The listing builds one solid part. Answer for the finished solid, in the listing's coordinates (mm). Face numbers are marked on the shaded views. Coordinates: 2 decimals unless noted, no trailing zeros. Order: outer loops, then holes, each group sorted by start corner. A loop starts at its lowest first (then second) coordinate and runs counter-clockwise, first axis right, second up. Notation, with made-up numbers: (-4, 56) -> (39, 56) arc R27 ccw to (39, 95) -> close; hole circle Ø9 at (-18.5, 52). An arc over 180 degrees is marked (long way). Answer in a Markdown table with one row per item.
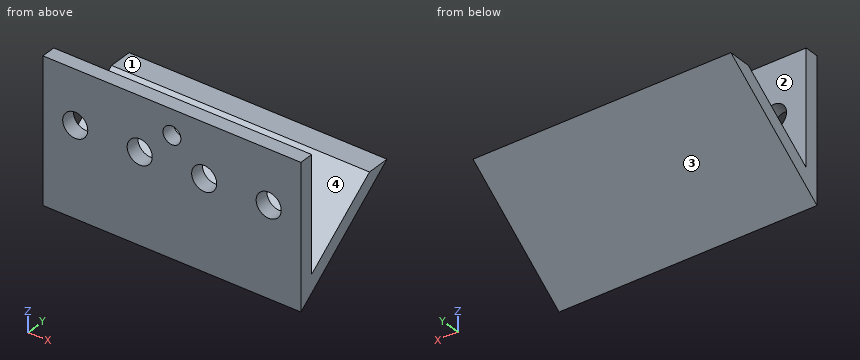
```python
from build123d import *

# Parameters (mm, degrees)
F0_W     = 72
F0_H     = 40
F0_R     = 3.5
F0_R_2   = 2.5
F1_DEPTH = 4
F3_DEPTH = 72
F5_DEPTH = 72


with BuildPart() as f1:
    # F0 (on Front) → F1 (new body)
    with BuildSketch(Plane.XZ):
        with Locations((0, -5)):
            Rectangle(F0_W, F0_H)
        with Locations((-27, 0)):
            Circle(F0_R, mode=Mode.SUBTRACT)
        with Locations((-9, 0)):
            Circle(F0_R, mode=Mode.SUBTRACT)
        with Locations((9, 0)):
            Circle(F0_R, mode=Mode.SUBTRACT)
        with Locations((27, 0)):
            Circle(F0_R, mode=Mode.SUBTRACT)
        with Locations((0, 8)):
            Circle(F0_R_2, mode=Mode.SUBTRACT)
    extrude(amount=F1_DEPTH)

    # F2 (on face) → F3 (cut)
    with BuildSketch(Plane.YZ.offset(36)):
        Polygon((0, -22), (-4, -25), (0, -25), align=None)
    extrude(amount=-F3_DEPTH, mode=Mode.SUBTRACT)

    # F4 (on face) → F5 (join)
    with BuildSketch(Plane.YZ.offset(36)):
        Polygon((0, -17), (0, -22), (28, -1), (21.5, -1), align=None)
    extrude(amount=-F5_DEPTH)


solid = f1.part
```
(1) A cutting plane is placed at A-A, the plane x = 0. Determine the outline of the cut face in (y, z), then the cut area to 3 significant figures.
Check values:
| item | result |
|---|---|
| outline | (-4, -25) -> (28, -1) -> (21.5, -1) -> (0, -17) -> (0, 5.5) -> (-4, 5.5) -> close; (-4, 10.5) -> (0, 10.5) -> (0, 15) -> (-4, 15) -> close |
| area | 256 mm² |
(2) Find the intervals of material crossed by line 1 along Y through (x, z) = (-24.5, 5); line 2 along Z through (x, y) = (27, -1); line 3 along Y through (x, z) = (6, -14), in increasing order. Write a range as from..to.
Check values:
| item | result |
|---|---|
| line 1 | -4..0 |
| line 2 | -22.75..-3.5, 3.5..15 |
| line 3 | -4..0, 4.03..10.67 |
(3) Flat-ended cylindrical pins translate along their axes: pin 1 (2 mm diameter, centred on x = 9, y = 16, fed in from +Z); pin 2 (9 mm diameter, centred on x = 27, z = 0, fed in from -Y); pin 3 (7 mm diameter, centred on x = -16, y = 26, fed in from +Z); pin 4 (8 mm diameter, centred on x = -17, y = 10, fed in from -Z). Find the tip coordinate at first contact, or state that the pin passes through.
Check values:
| item | result |
|---|---|
| pin 1 | z = -4.35 |
| pin 2 | y = -4 |
| pin 3 | z = -1 |
| pin 4 | z = -17.5 |
(4) A cutting plane is placed at C-C, the plane z = 8. Determine the outline of the cut face in (x, y), then the cut area to 3 significant figures.
Check values:
| item | result |
|---|---|
| outline | (-36, -4) -> (-2.5, -4) -> (-2.5, 0) -> (-36, 0) -> close; (2.5, -4) -> (36, -4) -> (36, 0) -> (2.5, 0) -> close |
| area | 268 mm² |
(5) A cutting plane is placed at D-D, the plane x = 27. Determine the outline of the cut face in (y, z).
Check values:
| item | result |
|---|---|
| outline | (-4, -25) -> (28, -1) -> (21.5, -1) -> (0, -17) -> (0, -3.5) -> (-4, -3.5) -> close; (-4, 3.5) -> (0, 3.5) -> (0, 15) -> (-4, 15) -> close |
(6) A cutting plane is placed at B-B, the plane z = 0. Determine the outline of the cut face in (x, y), then the cut area to 3 significant figures.
Check values:
| item | result |
|---|---|
| outline | (-36, -4) -> (-30.5, -4) -> (-30.5, 0) -> (-36, 0) -> close; (-23.5, -4) -> (-12.5, -4) -> (-12.5, 0) -> (-23.5, 0) -> close; (-5.5, -4) -> (5.5, -4) -> (5.5, 0) -> (-5.5, 0) -> close; (12.5, -4) -> (23.5, -4) -> (23.5, 0) -> (12.5, 0) -> close; (30.5, -4) -> (36, -4) -> (36, 0) -> (30.5, 0) -> close |
| area | 176 mm² |
(7) For a pull along Y with two mould halves and no side action, classify the marked faces 1, 2, 3 and 4 as released by +Y, released by -Y, zero draft, split by the parting line, or undercut.
Check values:
| item | result |
|---|---|
| face 1 | zero draft |
| face 2 | undercut |
| face 3 | released by +Y |
| face 4 | undercut |
